Autodesk Inventor part; units mm, degrees
ref_plane "YZ Plane" through (0, 0, 0) normal (1, 0, 0) x (0, 1, 0)
ref_plane "XZ Plane" through (0, 0, 0) normal (0, 1, 0) x (-1, 0, 0)
ref_plane "XY Plane" through (0, 0, 0) normal (0, 0, 1) x (1, 0, 0)
sketch "Sketch1" plane through (0, 0, 0) normal (0, 0, 1) x (1, 0, 0)
  point P0 (0, 0)
sketch "Sketch2" plane through (0, 0, 0) normal (0, 0, 1) x (1, 0, 0)
  arc A0 (0, 15.5) -> (0, -15.5) centre (0, 0) ccw
  line L0 (0, 0) -> (50, 0) construction
  line L1 (50, 0) -> (569.6152, 300) construction
  line L2 (569.6152, 300) -> (619.6152, 300) construction
  arc A1 (619.6152, 284.5) -> (619.6152, 315.5) centre (619.6152, 300) ccw
  line L3 (619.6152, 315.5) -> (566.5338, 315.5)
  line L4 (564.5338, 314.9641) -> (46.775, 16.0359)
  line L5 (44.775, 15.5) -> (0, 15.5)
  line L6 (619.6152, 284.5) -> (574.8403, 284.5)
  line L7 (572.8403, 283.9641) -> (55.0814, -14.9641)
  line L8 (53.0814, -15.5) -> (0, -15.5)
  line L9 (46.641, 16.5359) -> (564.3999, 315.4641)
  line L10 (566.3999, 316) -> (619.6152, 316)
  arc A2 (619.6152, 284) -> (619.6152, 316) centre (619.6152, 300) ccw
  line L11 (619.6152, 284) -> (574.9742, 284)
  line L12 (572.9742, 283.4641) -> (55.2154, -15.4641)
  line L13 (53.2154, -16) -> (0, -16)
  arc A3 (0, 16) -> (0, -16) centre (0, 0) ccw
  line L14 (0, 16) -> (44.641, 16)
  line L15 (0, 15) -> (44.909, 15)
  line L16 (46.909, 15.5359) -> (564.6678, 314.4641)
  line L17 (566.6678, 315) -> (619.6152, 315)
  arc A4 (619.6152, 285) -> (619.6152, 315) centre (619.6152, 300) ccw
  line L18 (619.6152, 285) -> (574.7063, 285)
  line L19 (572.7063, 284.4641) -> (54.9474, -14.4641)
  line L20 (52.9474, -15) -> (0, -15)
  arc A5 (0, 15) -> (0, -15) centre (0, 0) ccw
  arc A6 (44.641, 16) -> (46.641, 16.5359) centre (44.641, 20) ccw
  arc A7 (44.775, 15.5) -> (46.775, 16.0359) centre (44.775, 19.5) ccw
  arc A8 (44.909, 15) -> (46.909, 15.5359) centre (44.909, 19) ccw
  arc A9 (52.9474, -15) -> (54.9474, -14.4641) centre (52.9474, -11) ccw
  arc A10 (53.0814, -15.5) -> (55.0814, -14.9641) centre (53.0814, -11.5) ccw
  arc A11 (53.2154, -16) -> (55.2154, -15.4641) centre (53.2154, -12) ccw
  arc A12 (574.7063, 285) -> (572.7063, 284.4641) centre (574.7063, 281) ccw
  arc A13 (574.8403, 284.5) -> (572.8403, 283.9641) centre (574.8403, 280.5) ccw
  arc A14 (574.9742, 284) -> (572.9742, 283.4641) centre (574.9742, 280) ccw
  arc A15 (566.3999, 316) -> (564.3999, 315.4641) centre (566.3999, 312) ccw
  arc A16 (566.5338, 315.5) -> (564.5338, 314.9641) centre (566.5338, 311.5) ccw
  arc A17 (566.6678, 315) -> (564.6678, 314.4641) centre (566.6678, 311) ccw
  dimension "d0" = 31
  dimension "d1" = 50
  dimension "d2" = 600
  dimension "d3" = 150
  dimension "d4" = 50
  dimension "d5" = 31
  dimension "d6" = 4
  dimension "d7" = 4
  dimension "d8" = 4
  dimension "d9" = 4
  dimension "d10" = 4
  dimension "d11" = 4
  dimension "d12" = 4
  dimension "d13" = 4
  dimension "d14" = 4
  dimension "d15" = 4
extrude "Extrusion1" add sketch "Sketch2" along normal blind 43 contours L5 A7 L4 A16 L3 A1 L6 A13 L7 A10 L8 A0 | L9 A15 L10 A2 L11 A14 L12 A11 L13 A3 L14 A6
properties part number "Assembly belt For lifting"
Verification items for the finished model (mm, model axes). A direction names the side the tool comes from. Round coordinates to 2 decimals unless told otherwise and drop trailing zeros. Write each loop counter-clockwise with the first axis right and the second up, starting at its lowest first coordinate (ties: lowest second). Pieces come first, ordered by that corner, then holes. Notation, with made-up numbers: (-19.75, -18) - (39.25, -18) arc R18 ccw to (39.25, -5) - close; hole circle Ø4 at (89, 37.25). An arc over 180 degrees is marked (long way). Answer as a JSON object with one key per item and string values. Group by question number.
Q1. Mould release check, pull along X, two halves, no side actions. Record for faces 4 (the flat face through (598, 284, 21)), 5 (the cylindrical face through (635.61, 300.35, 21.2)), 6 (the flat face through (593, 315, 21)), 7 (the cylindrical face through (-16, 0, 21)): released by +X, released by -X, zero draft, split by the parting line, or undercut.
Q2. Section check A-A, the plane z = 30. Enter the section's corners in (x, y).
Q3. Section check C-C, the plane x = 340.5. Enter the section's corners in (y, z), plus the area to 3 significant figures.
Q4. Section check B-B, the plane y = 142.5. Enter the section's corners in (x, z), plus the area to 3 significant figures.
Q5. Go/stop test with flat-tipped pins: pin 1 Ø12 at (y, z) = (243, 8) entering from -X; pin 2 Ø1.5 at (x, z) = (330.5, 16.5) entering from -Y; pin 3 Ø1.5 at (x, z) = (80.5, 30) entering from -Y. Record where each tip stops, or that it passes through.
Q6. Thickness scan on line 1 (Y direction, x = 23, z = 4.5); line 2 (Y direction, x = 323, z = 32.5); line 3 (X direction, y = 89, z = 24.5). Record the ranges inside material, lowest first.
Q7. Tool access check on faces 1 (the flat face through (27, -16, 21)), 2 (the flat face through (22, 16, 21)), 3 (the flat face through (27, -15, 21)). Record the directions out of +Z, -Z, +X, -X, +Y, -Y that give a thin tool (end or side, any length) a straight path to the whole face; none if there is none.
Found:
{
 "1": {"face 4": "zero draft", "face 5": "released by +X", "face 6": "undercut", "face 7": "released by -X"},
 "2": {"outline": "(0, -16) - (53.22, -16) arc R4 ccw to (55.22, -15.46) - (572.97, 283.46) arc R4 cw to (574.97, 284) - (619.62, 284) arc R16 ccw to (619.62, 316) - (566.4, 316) arc R4 ccw to (564.4, 315.46) - (46.64, 16.54) arc R4 cw to (44.64, 16) - (0, 16) arc R16 ccw to start; hole (0, -15) - (52.95, -15) arc R4 ccw to (54.95, -14.46) - (572.71, 284.46) arc R4 cw to (574.71, 285) - (619.62, 285) arc R15 ccw to (619.62, 315) - (566.67, 315) arc R4 ccw to (564.67, 314.46) - (46.91, 15.54) arc R4 cw to (44.91, 15) - (0, 15) arc R15 ccw to start"},
 "3": {"outline": "(149.25, 0) - (150.4, 0) - (150.4, 43) - (149.25, 43) - close; (185.04, 0) - (186.2, 0) - (186.2, 43) - (185.04, 43) - close", "area": "99.3 mm^2"},
 "4": {"outline": "(264.82, 0) - (266.82, 0) - (266.82, 43) - (264.82, 43) - close; (326.82, 0) - (328.82, 0) - (328.82, 43) - (326.82, 43) - close", "area": "172 mm^2"},
 "5": {"pin 1": "stops at x = 428.5", "pin 2": "stops at y = 143.04", "pin 3": "stops at y = -1.3"},
 "6": {"line 1": "y = -16 to -15, 15 to 16", "line 2": "y = 139.14 to 140.3, 174.94 to 176.09", "line 3": "x = 172.15 to 174.15, 234.15 to 236.15"},
 "7": {"face 1": "+Z, -Z, +X, -X, -Y", "face 2": "+Z, -Z, -X, +Y", "face 3": "+Z, -Z"}
}
